```python
from build123d import *

# Parameters (mm, degrees)
ESQUISSE1_W        = 71.7
ESQUISSE1_H        = 52.8
BOSS_EXTRU_1_DEPTH = 7.3
ESQUISSE2_R        = 0.85
BOSS_EXTRU_2_DEPTH = 20


with BuildPart() as part:
    # Esquisse1 → Boss.-Extru.1 (new, symmetric)
    with BuildSketch(Plane(origin=(0, 0, 0), x_dir=(1, 0, 0), z_dir=(0, 1, 0))):
        Rectangle(ESQUISSE1_W, ESQUISSE1_H)
    extrude(amount=BOSS_EXTRU_1_DEPTH, both=True)

    # Esquisse2 → Boss.-Extru.2 (add)
    with BuildSketch(Plane.ZY.offset(35.85)):
        with Locations(Location((-24.787698277, 1.136553851, 0), (0, 0, 180))):
            Circle(ESQUISSE2_R)
        with Locations(Location((-24.787698277, -1.136553851, 0), (0, 0, 180))):
            Circle(ESQUISSE2_R)
    extrude(amount=BOSS_EXTRU_2_DEPTH)


solid = part.part
```
Model file for the job. Use its own axes, mm. A direction names the side the tool comes from. Round coordinates to 2 decimals unless told otherwise and drop trailing zeros. Write each loop counter-clockwise with the first axis right and the second up, starting at its lowest first coordinate (ties: lowest second). Pieces come first, ordered by that corner, then holes. Notation, with made-up numbers: (33.5, 23.25) - (90.5, 23.25) arc R18 ccw to (90.5, 34.25) - close; hole circle Ø3 at (20.5, 14.25). An arc over 180 degrees is marked (long way). Use CSV: the item, a comma, the result in double quotes. Start each with the question number.
Item 1: Pin check, flat tips, straight feed: P1, Ø6, axis at x = -38.5, y = 3, coming from the -Z side; P2, Ø4.5, axis at y = 1, z = 4.5, coming from the -X side. Stop position of each tip, or through.
Item 2: Drill centre line: L1, parallel to X at y = -4.5, z = -16. Where is it in solid material? Low to high. Write a range as [from, to].
Item 3: Band-saw the part on A-A (y = -5). Write the cut outline in (x, z), and give its area (3 significant figures).
Item 4: Tool access for faces 1 (the face through (-55.85, 1, -25)), 2 (the face through (-45.71, 1.1, -23.94)): list every direction of +Z, -Z, +X, -X, +Y, -Y with a clear straight run to the whole face (end or side of a thin tool).
Item 5: Two-plate mould, pull along Y, no slides. Class faces 3 (the face through (-1, 7.3, 0)), 4 (the face through (-55.85, -1, -25)), 5 (the face through (-45.71, -1.17, -23.94)), 6 (the face through (-1, -7.3, 0)): released by +Y, released by -Y, zero draft, split by the parting line, or undercut.
Item 6: Band-saw the part on B-B (z = 20). Write the cut outline in (x, y), and give its area (3 significant figures).
Checked values:
1,P1,"stops at z = -26.4"
1,P2,"stops at x = -35.85"
2,L1,"x = [-35.85, 35.85]"
3,outline,"(-35.85, -26.4) - (35.85, -26.4) - (35.85, 26.4) - (-35.85, 26.4) - close"
3,area,"3,790 mm²"
4,face 1,"+Z, -Z, -X, +Y, -Y"
4,face 2,"-X"
5,face 3,"released by +Y"
5,face 4,"zero draft"
5,face 5,"undercut"
5,face 6,"released by -Y"
6,outline,"(-35.85, -7.3) - (35.85, -7.3) - (35.85, 7.3) - (-35.85, 7.3) - close"
6,area,"1,050 mm²"
